from build123d import *

# Parameters (mm, degrees)
F2_DEPTH       = 7
F5_D           = 3.1
F5_CSINK_D     = 6
F5_CSINK_ANGLE = 90
F6_D           = 3.1
F6_CSINK_D     = 6
F6_CSINK_ANGLE = 90


with BuildPart() as f2:
    # F1 (on Front) → F2 (new body)
    with BuildSketch(Plane.XZ):
        with BuildLine():
            Line((-6.05, 1.15), (0, 1.15))
            Line((0, 1.15), (6.05, 1.15))
            Line((6.05, 1.15), (6.05, 0))
            Line((6.05, 0), (8.05, 0))
            Line((8.05, 0), (8.05, 1.15))
            Line((8.05, 1.15), (20.15, 1.15))
            Line((20.15, 1.15), (20.15, 0))
            Line((20.15, 0), (26.65, 0))
            Line((26.65, 0), (26.65, 2.05))
            ThreePointArc((26.65, 2.05), (26.4742640687, 2.4742640687), (26.05, 2.65))
            Line((26.05, 2.65), (0, 2.65))
            Line((0, 2.65), (-26.05, 2.65))
            ThreePointArc((-26.05, 2.65), (-26.4742640687, 2.4742640687), (-26.65, 2.05))
            Line((-26.65, 2.05), (-26.65, 0))
            Line((-26.65, 0), (-20.15, 0))
            Line((-20.15, 0), (-20.15, 1.15))
            Line((-20.15, 1.15), (-8.05, 1.15))
            Line((-8.05, 1.15), (-8.05, 0))
            Line((-8.05, 0), (-6.05, 0))
            Line((-6.05, 0), (-6.05, 1.15))
        make_face()
    extrude(amount=F2_DEPTH)

    # F5 (through all)
    with Locations(Plane.XY.offset(2.65)):
        with Locations((-23.4, -3.5)):
            CounterSinkHole(F5_D / 2, F5_CSINK_D / 2, counter_sink_angle=F5_CSINK_ANGLE)

    # F6 (through all)
    with Locations(Plane.XY.offset(2.65)):
        with Locations((23.4, -3.5)):
            CounterSinkHole(F6_D / 2, F6_CSINK_D / 2, counter_sink_angle=F6_CSINK_ANGLE)


solid = f2.part
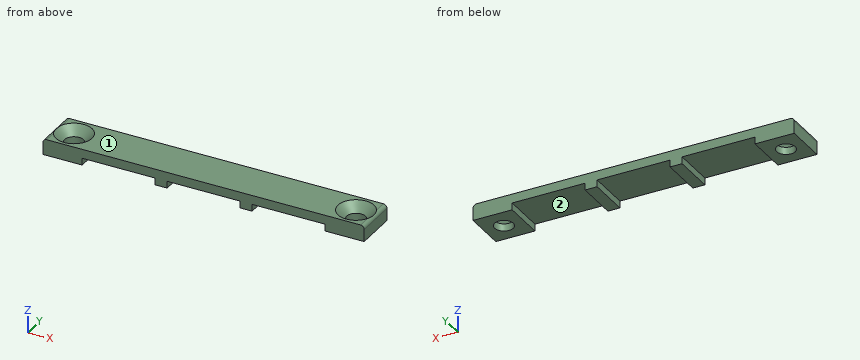
Input: part model. Units: mm. Frame: model coordinates. Face numbers are marked on the shaded views. A direction names the side the tool comes from. Round coordinates to 2 decimals unless told otherwise and drop trailing zeros. Write each loop counter-clockwise with the first axis right and the second up, starting at its lowest first coordinate (ties: lowest second). Pieces come first, ordered by that corner, then holes.
1) Cut plane A-A (x = 23.4). Return the cut outline in (y, z).
2) Contact query for flat-ended pins moving along their axis: P1, Ø2, axis at x = -11.5, y = -5, coming from the -Z side; P2, Ø1.9, axis at x = 23.4, y = -3.5, coming from the -Z side. Output: stop coordinate, or through.
3) Ray query, L1, parallel to X at y = -0.75, z = 0.4; L2, parallel to X at y = -3.5, z = 0.95; L3, parallel to Y at x = 23.4, z = 0.85. Return the intervals inside material, ascending.
4) Reachability of the marked faces 1 and 2 from +Z, -Z, +X, -X, +Y, -Y: full face, straight path, thin tool, end or side. Return the list, or none.
5) Cut plane B-B (y = -3.5). Return the cut outline in (x, z), then the cut area to 3 significant figures.
Geometry says:
1. outline: (-7, 0) - (-5.05, 0) - (-5.05, 1.2) - (-6.5, 2.65) - (-7, 2.65) - close; (-1.95, 0) - (0, 0) - (0, 2.65) - (-0.5, 2.65) - (-1.95, 1.2) - close
2. P1: stops at z = 1.15
2. P2: passes through
3. L1: x = -26.65 to -20.15, -8.05 to -6.05, 6.05 to 8.05, 20.15 to 26.65
3. L2: x = -26.65 to -24.95, -21.85 to -20.15, -8.05 to -6.05, 6.05 to 8.05, 20.15 to 21.85, 24.95 to 26.65
3. L3: y = -7 to -5.05, -1.95 to 0
4. face 1: +Z, +X, -X, +Y, -Y
4. face 2: -Z, +Y, -Y
5. outline: (-26.65, 0) - (-24.95, 0) - (-24.95, 1.2) - (-26.33, 2.58) arc R0.6 ccw to (-26.65, 2.05) - close; (-21.85, 0) - (-20.15, 0) - (-20.15, 1.15) - (-8.05, 1.15) - (-8.05, 0) - (-6.05, 0) - (-6.05, 1.15) - (6.05, 1.15) - (6.05, 0) - (8.05, 0) - (8.05, 1.15) - (20.15, 1.15) - (20.15, 0) - (21.85, 0) - (21.85, 1.2) - (20.4, 2.65) - (-20.4, 2.65) - (-21.85, 1.2) - close; (24.95, 0) - (26.65, 0) - (26.65, 2.05) arc R0.6 ccw to (26.33, 2.58) - (24.95, 1.2) - close
5. area: 78.7 mm2
